The model under review builds one solid part; all positions refer to its coordinate system, in mm. A direction names the side the tool comes from. Coordinates: 2 decimals unless noted, no trailing zeros. Write each loop counter-clockwise with the first axis right and the second up, starting at its lowest first coordinate (ties: lowest second). Pieces come first, ordered by that corner, then holes.
1) Add section C-C, the plane y = 8.5. State the section outline as (x, z) points, then the cut area to 3 significant figures.
2) Machinability: for faces 1 (the flat face through (126, 33.714, 14)), 2 (the flat face through (126, 37.714, 15)), which of the approach directions +Z, -Z, +X, -X, +Y, -Y give a long, thin tool a straight path to every point of the face, cutting with its end or side? Answer none if there is none.
3) Mouldability with a two-part tool opening along Y and no side actions: class faces 3 (the flat face through (126, -137.286, 15)), 4 (the flat face through (126, -133.286, 14)), 5 (the flat face through (126, -49, 30)) as released by +Y, released by -Y, zero draft, split by the parting line, or undercut.
4) For P1, Ø10, axis at x = 233.5, y = -47.5, coming from the -Z side, flat-tipped, find the tip position at first contact; note if it passes through.
5) For line 1 (X direction, y = -112, z = 4.25); line 2 (Y direction, x = 70.5, z = 4.75); line 3 (Z direction, x = 93.5, y = 24), list the stretches that pass through material, from the lowest coordinate up.
6) Add section A-A, the plane z = 17.5. State the section outline as (x, y) points.
7) Add section B-B, the plane x = 178.5. State the section outline as (y, z) points.
from build123d import *

# Parameters (mm, degrees)
F0_W         = 370
F0_H         = 175
F1_DEPTH     = 30
F2_T         = -4
F3_R         = 1.5
F4_T1_DEPTH  = 172
F4_T3_DEPTH  = 27
F4_T5_DEPTH  = 367
F4_S9_W      = 1.5
F4_S9_H      = 1.5
F4_T10_DEPTH = 1.5
F4_S15_W     = 1.5
F4_S15_H     = 1.5
F4_T16_DEPTH = 1.5
F4_S21_W     = 1.5
F4_S21_H     = 1.5
F4_T22_DEPTH = 1.5
F4_S27_W     = 1.5
F4_S27_H     = 1.5
F4_T28_DEPTH = 1.5
F4_S33_W     = 1.5
F4_S33_H     = 1.5
F4_T34_DEPTH = 1.5
F4_S39_W     = 1.5
F4_S39_H     = 1.5
F4_T40_DEPTH = 1.5
F4_S45_W     = 1.5
F4_S45_H     = 1.5
F4_T46_DEPTH = 1.5
F4_S51_W     = 1.5
F4_S51_H     = 1.5
F4_T52_DEPTH = 1.5


# Not quite as in the source:
# - a fillet or chamfer that OpenCascade refuses, or shapes differently, is made with other operations: its cross-section is extruded or revolved along the edge and cut away or added


with BuildPart() as f1:
    # F0 (on Top) → F1 (new body)
    with BuildSketch(Plane.XY):
        with Locations((128.3509446681, -49.7856229544)):
            Rectangle(F0_W, F0_H)
    extrude(amount=F1_DEPTH)

    # F2
    f2_openings = [f1.faces().sort_by_distance(p)[0] for p in [
        (128.350945, -49.785623, 0),
    ]]
    offset(amount=F2_T, openings=f2_openings)

    # F3
    f3_edges = [f1.edges().sort_by_distance(p)[0] for p in [
        (128.350945, -137.285623, 0),
        (-56.649055, -49.785623, 0),
        (-52.649055, -49.785623, 0),
        (128.350945, -133.285623, 0),
        (128.350945, 37.714377, 0),
        (128.350945, 33.714377, 0),
        (309.350945, -49.785623, 0),
        (313.350945, -49.785623, 0),
    ]]
    fillet(f3_edges, radius=F3_R)

    # F4: fillet of radius 1.5 on 8 edges, made by hand

    # F4_s2 → F4_t1 (cut)
    with BuildSketch(Plane.XZ.offset(-36.2143770456)):
        with BuildLine():
            ThreePointArc((-55.1490553319, 30), (-56.2097155037, 29.5606601718), (-56.6490553319, 28.5))
            Line((-56.6490553319, 28.5), (-56.6490553319, 30))
            Line((-56.6490553319, 30), (-55.1490553319, 30))
        make_face()
        with BuildLine():
            ThreePointArc((313.3509446681, 28.5), (312.9116048398, 29.5606601718), (311.8509446681, 30))
            Line((311.8509446681, 30), (313.3509446681, 30))
            Line((313.3509446681, 30), (313.3509446681, 28.5))
        make_face()
    extrude(amount=F4_T1_DEPTH, mode=Mode.SUBTRACT)

    # F4_s4 → F4_t3 (cut)
    with BuildSketch(Plane.XY.offset(1.5)):
        with BuildLine():
            ThreePointArc((-55.1490553319, 37.7143770456), (-56.2097155037, 37.2750372174), (-56.6490553319, 36.2143770456))
            Line((-56.6490553319, 36.2143770456), (-56.6490553319, 37.7143770456))
            Line((-56.6490553319, 37.7143770456), (-55.1490553319, 37.7143770456))
        make_face()
        with BuildLine():
            ThreePointArc((-56.6490553319, -135.7856229544), (-56.2097155037, -136.8462831261), (-55.1490553319, -137.2856229544))
            Line((-55.1490553319, -137.2856229544), (-56.6490553319, -137.2856229544))
            Line((-56.6490553319, -137.2856229544), (-56.6490553319, -135.7856229544))
        make_face()
        with BuildLine():
            ThreePointArc((313.3509446681, -135.7856229544), (312.9116048398, -136.8462831261), (311.8509446681, -137.2856229544))
            Line((311.8509446681, -137.2856229544), (313.3509446681, -137.2856229544))
            Line((313.3509446681, -137.2856229544), (313.3509446681, -135.7856229544))
        make_face()
        with BuildLine():
            ThreePointArc((311.8509446681, 37.7143770456), (312.9116048398, 37.2750372174), (313.3509446681, 36.2143770456))
            Line((313.3509446681, 36.2143770456), (313.3509446681, 37.7143770456))
            Line((313.3509446681, 37.7143770456), (311.8509446681, 37.7143770456))
        make_face()
    extrude(amount=F4_T3_DEPTH, mode=Mode.SUBTRACT)

    # F4_s6 → F4_t5 (cut)
    with BuildSketch(Plane.YZ.offset(-55.1490553319)):
        with BuildLine():
            ThreePointArc((-135.7856229544, 30), (-136.8462831261, 29.5606601718), (-137.2856229544, 28.5))
            Line((-137.2856229544, 28.5), (-137.2856229544, 30))
            Line((-137.2856229544, 30), (-135.7856229544, 30))
        make_face()
        with BuildLine():
            ThreePointArc((37.7143770456, 28.5), (37.2750372174, 29.5606601718), (36.2143770456, 30))
            Line((36.2143770456, 30), (37.7143770456, 30))
            Line((37.7143770456, 30), (37.7143770456, 28.5))
        make_face()
    extrude(amount=F4_T5_DEPTH, mode=Mode.SUBTRACT)


with BuildPart() as f4_tool8:
    # F4_s9 → F4_t10 (new body)
    with BuildSketch(Plane.XZ.offset(-36.2143770456)):
        with Locations((312.6009446681, 0.75)):
            Rectangle(F4_S9_W, F4_S9_H)
    extrude(amount=-F4_T10_DEPTH)

    # F4_s11 → F4_t12 (revolve, cut)
    with BuildSketch(Plane(origin=(311.8509446681, 36.2143770456, 1.5), x_dir=(-0.7071067812, 0, 0.7071067812), z_dir=(-0.7071067812, 0, -0.7071067812))):
        with BuildLine():
            ThreePointArc((0, -1.5), (1.5, 0), (0, 1.5))
            Line((0, 1.5), (0, -1.5))
        make_face()
    revolve(axis=Axis((311.8509446681, 36.2143770456, 1.5), (0, 1, 0)), mode=Mode.SUBTRACT)


with BuildPart() as f1_1:
    add(f1.part)

    # F4_t7: cut F4_tool8
    add(f4_tool8.part, mode=Mode.SUBTRACT)


with BuildPart() as f4_tool14:
    # F4_s15 → F4_t16 (new body)
    with BuildSketch(Plane.YZ.offset(311.8509446681)):
        with Locations((-136.5356229544, 0.75)):
            Rectangle(F4_S15_W, F4_S15_H)
    extrude(amount=F4_T16_DEPTH)

    # F4_s17 → F4_t18 (revolve, cut)
    with BuildSketch(Plane(origin=(311.8509446681, -135.7856229544, 1.5), x_dir=(0, 0.7071067812, 0.7071067812), z_dir=(0, 0.7071067812, -0.7071067812))):
        with BuildLine():
            ThreePointArc((0, -1.5), (1.5, 0), (0, 1.5))
            Line((0, 1.5), (0, -1.5))
        make_face()
    revolve(axis=Axis((311.8509446681, -135.7856229544, 1.5), (1, 0, 0)), mode=Mode.SUBTRACT)


with BuildPart() as f1_2:
    add(f1_1.part)

    # F4_t13: cut F4_tool14
    add(f4_tool14.part, mode=Mode.SUBTRACT)


with BuildPart() as f4_tool20:
    # F4_s21 → F4_t22 (new body)
    with BuildSketch(Plane.YZ.offset(-55.1490553319)):
        with Locations((-136.5356229544, 0.75)):
            Rectangle(F4_S21_W, F4_S21_H)
    extrude(amount=-F4_T22_DEPTH)

    # F4_s23 → F4_t24 (revolve, cut)
    with BuildSketch(Plane(origin=(-55.1490553319, -135.7856229544, 1.5), x_dir=(0, 0.7071067812, 0.7071067812), z_dir=(0, -0.7071067812, 0.7071067812))):
        with BuildLine():
            ThreePointArc((0, -1.5), (1.5, 0), (0, 1.5))
            Line((0, 1.5), (0, -1.5))
        make_face()
    revolve(axis=Axis((-55.1490553319, -135.7856229544, 1.5), (-1, 0, 0)), mode=Mode.SUBTRACT)


with BuildPart() as f1_3:
    add(f1_2.part)

    # F4_t19: cut F4_tool20
    add(f4_tool20.part, mode=Mode.SUBTRACT)


with BuildPart() as f4_tool26:
    # F4_s27 → F4_t28 (new body)
    with BuildSketch(Plane.XZ.offset(-36.2143770456)):
        with Locations((-55.8990553319, 0.75)):
            Rectangle(F4_S27_W, F4_S27_H)
    extrude(amount=-F4_T28_DEPTH)

    # F4_s29 → F4_t30 (revolve, cut)
    with BuildSketch(Plane(origin=(-55.1490553319, 36.2143770456, 1.5), x_dir=(0.7071067812, 0, 0.7071067812), z_dir=(-0.7071067812, 0, 0.7071067812))):
        with BuildLine():
            ThreePointArc((0, -1.5), (1.5, 0), (0, 1.5))
            Line((0, 1.5), (0, -1.5))
        make_face()
    revolve(axis=Axis((-55.1490553319, 36.2143770456, 1.5), (0, 1, 0)), mode=Mode.SUBTRACT)


with BuildPart() as f1_4:
    add(f1_3.part)

    # F4_t25: cut F4_tool26
    add(f4_tool26.part, mode=Mode.SUBTRACT)


with BuildPart() as f4_tool32:
    # F4_s33 → F4_t34 (new body)
    with BuildSketch(Plane.XZ.offset(-36.2143770456)):
        with Locations((-55.8990553319, 29.25)):
            Rectangle(F4_S33_W, F4_S33_H)
    extrude(amount=-F4_T34_DEPTH)

    # F4_s35 → F4_t36 (revolve, cut)
    with BuildSketch(Plane(origin=(-55.1490553319, 36.2143770456, 28.5), x_dir=(0.7071067812, 0, -0.7071067812), z_dir=(0.7071067812, 0, 0.7071067812))):
        with BuildLine():
            ThreePointArc((0, -1.5), (1.5, 0), (0, 1.5))
            Line((0, 1.5), (0, -1.5))
        make_face()
    revolve(axis=Axis((-55.1490553319, 36.2143770456, 28.5), (0, 1, 0)), mode=Mode.SUBTRACT)


with BuildPart() as f1_5:
    add(f1_4.part)

    # F4_t31: cut F4_tool32
    add(f4_tool32.part, mode=Mode.SUBTRACT)


with BuildPart() as f4_tool38:
    # F4_s39 → F4_t40 (new body)
    with BuildSketch(Plane.XY.offset(28.5)):
        with Locations((-55.8990553319, -136.5356229544)):
            Rectangle(F4_S39_W, F4_S39_H)
    extrude(amount=F4_T40_DEPTH)

    # F4_s41 → F4_t42 (revolve, cut)
    with BuildSketch(Plane(origin=(-55.1490553319, -135.7856229544, 28.5), x_dir=(0.7071067812, 0.7071067812, 0), z_dir=(0.7071067812, -0.7071067812, 0))):
        with BuildLine():
            ThreePointArc((0, -1.5), (1.5, 0), (0, 1.5))
            Line((0, 1.5), (0, -1.5))
        make_face()
    revolve(axis=Axis((-55.1490553319, -135.7856229544, 28.5), (0, 0, 1)), mode=Mode.SUBTRACT)


with BuildPart() as f1_6:
    add(f1_5.part)

    # F4_t37: cut F4_tool38
    add(f4_tool38.part, mode=Mode.SUBTRACT)


with BuildPart() as f4_tool44:
    # F4_s45 → F4_t46 (new body)
    with BuildSketch(Plane.YZ.offset(311.8509446681)):
        with Locations((-136.5356229544, 29.25)):
            Rectangle(F4_S45_W, F4_S45_H)
    extrude(amount=F4_T46_DEPTH)

    # F4_s47 → F4_t48 (revolve, cut)
    with BuildSketch(Plane(origin=(311.8509446681, -135.7856229544, 28.5), x_dir=(0, 0.7071067812, -0.7071067812), z_dir=(0, -0.7071067812, -0.7071067812))):
        with BuildLine():
            ThreePointArc((0, -1.5), (1.5, 0), (0, 1.5))
            Line((0, 1.5), (0, -1.5))
        make_face()
    revolve(axis=Axis((311.8509446681, -135.7856229544, 28.5), (1, 0, 0)), mode=Mode.SUBTRACT)


with BuildPart() as f1_7:
    add(f1_6.part)

    # F4_t43: cut F4_tool44
    add(f4_tool44.part, mode=Mode.SUBTRACT)


with BuildPart() as f4_tool50:
    # F4_s51 → F4_t52 (new body)
    with BuildSketch(Plane.XZ.offset(-36.2143770456)):
        with Locations((312.6009446681, 29.25)):
            Rectangle(F4_S51_W, F4_S51_H)
    extrude(amount=-F4_T52_DEPTH)

    # F4_s53 → F4_t54 (revolve, cut)
    with BuildSketch(Plane(origin=(311.8509446681, 36.2143770456, 28.5), x_dir=(-0.7071067812, 0, -0.7071067812), z_dir=(0.7071067812, 0, -0.7071067812))):
        with BuildLine():
            ThreePointArc((0, -1.5), (1.5, 0), (0, 1.5))
            Line((0, 1.5), (0, -1.5))
        make_face()
    revolve(axis=Axis((311.8509446681, 36.2143770456, 28.5), (0, 1, 0)), mode=Mode.SUBTRACT)


with BuildPart() as f1_8:
    add(f1_7.part)

    # F4_t49: cut F4_tool50
    add(f4_tool50.part, mode=Mode.SUBTRACT)


solid = f1_8.part
Geometry results:
1. outline: (-56.65, 1.5) arc R1.5 ccw to (-55.15, 0) - (-54.15, 0) arc R1.5 ccw to (-52.65, 1.5) - (-52.65, 26) - (309.35, 26) - (309.35, 1.5) arc R1.5 ccw to (310.85, 0) - (311.85, 0) arc R1.5 ccw to (313.35, 1.5) - (313.35, 28.5) arc R1.5 ccw to (311.85, 30) - (-55.15, 30) arc R1.5 ccw to (-56.65, 28.5) - close
1. area: 1,690 mm2
2. face 1: -Z
2. face 2: +Z, -Z, +X, -X, +Y
3. face 3: released by -Y
3. face 4: undercut
3. face 5: zero draft
4. P1: stops at z = 26
5. line 1: x = -56.65 to -52.65, 309.35 to 313.35
5. line 2: y = -137.29 to -133.29, 33.71 to 37.71
5. line 3: z = 26 to 30
6. outline: (-56.65, -135.79) arc R1.5 ccw to (-55.15, -137.29) - (311.85, -137.29) arc R1.5 ccw to (313.35, -135.79) - (313.35, 36.21) arc R1.5 ccw to (311.85, 37.71) - (-55.15, 37.71) arc R1.5 ccw to (-56.65, 36.21) - close; hole (-52.65, -133.29) - (309.35, -133.29) - (309.35, 33.71) - (-52.65, 33.71) - close
7. outline: (-137.29, 1.5) arc R1.5 ccw to (-135.79, 0) - (-134.79, 0) arc R1.5 ccw to (-133.29, 1.5) - (-133.29, 26) - (33.71, 26) - (33.71, 1.5) arc R1.5 ccw to (35.21, 0) - (36.21, 0) arc R1.5 ccw to (37.71, 1.5) - (37.71, 28.5) arc R1.5 ccw to (36.21, 30) - (-135.79, 30) arc R1.5 ccw to (-137.29, 28.5) - close
